Work out the finished part from the listing and answer in its coordinate system (mm). Give positions to 0.01 mm unless a question says otherwise; leave off trailing zeros. Order: outer loops, then holes, each group sorted by start corner. A loop starts at its lowest first (then second) coordinate and runs counter-clockwise, first axis right, second up. Notation, with made-up numbers: (-9, -23) - (23, -23) arc R16 cw to (23, -4) - close; hole circle Ø6 at (54.5, -15.75). An arc over 180 degrees is marked (long way). Put each result on its own line as item: value.
```python
from build123d import *

# Parameters (mm, degrees)
F0_R     = 300
F0_R_2   = 2.25
F0_R_3   = 50
F1_DEPTH = 18


with BuildPart() as f1:
    # F0 (on Top) → F1 (new body)
    with BuildSketch(Plane.XY):
        Circle(F0_R)
        with Locations((-65, -80)):
            Circle(F0_R_2, mode=Mode.SUBTRACT)
        with Locations((-40, -80)):
            Circle(F0_R_2, mode=Mode.SUBTRACT)
        with Locations((40, -80)):
            Circle(F0_R_2, mode=Mode.SUBTRACT)
        with Locations((65, -80)):
            Circle(F0_R_2, mode=Mode.SUBTRACT)
        with Locations((-65, 270)):
            Circle(F0_R_2, mode=Mode.SUBTRACT)
        with Locations((-40, 270)):
            Circle(F0_R_2, mode=Mode.SUBTRACT)
        Circle(F0_R_3, mode=Mode.SUBTRACT)
        with Locations((40, 270)):
            Circle(F0_R_2, mode=Mode.SUBTRACT)
        with Locations((65, 270)):
            Circle(F0_R_2, mode=Mode.SUBTRACT)
    extrude(amount=F1_DEPTH)


solid = f1.part
```
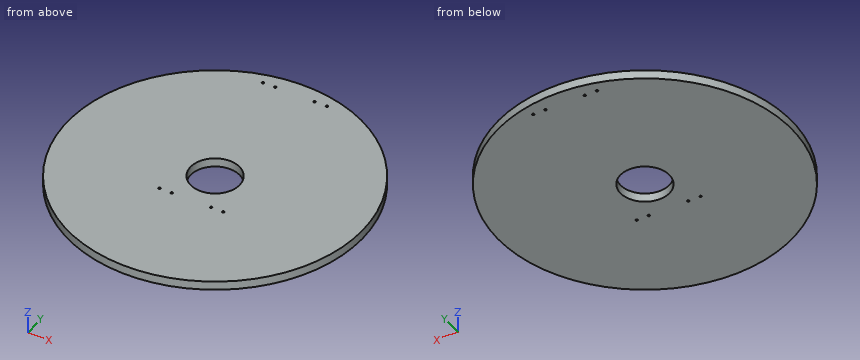
(1) Straight lines are drawn through the part: line 1 (Y direction, x = -40, z = 12.75); line 2 (Y direction, x = 65, z = 9.5); line 3 (Y direction, x = -42.5, z = 9.25). For each, find the intervals that lie inside material, in ascending order.
Geometry check:
line 1: y = -297.32 to -82.25, -77.75 to -30, 30 to 267.75, 272.25 to 297.32
line 2: y = -292.87 to -82.25, -77.75 to 267.75, 272.25 to 292.87
line 3: y = -296.97 to -26.34, 26.34 to 296.97
(2) Section D-D, the plane x = -115.5 is taken. Write down the section's boundary in (y, z), then the cut area to 3 significant figures.
Geometry check:
outline: (-276.87, 0) - (276.87, 0) - (276.87, 18) - (-276.87, 18) - close
area: 9,970 mm²
(3) Section C-C, the plane z = 5.75 is taken. Count the separate pieces of the cut face and the enclosed holes in it, then the cut area to 3 significant figures.
Geometry check:
separate pieces: 1
enclosed holes: 9
area: 275,000 mm²
(4) Section A-A, the plane y = 0 is taken. Write down the section's boundary in (x, z).
Geometry check:
outline: (-300, 0) - (-50, 0) - (-50, 18) - (-300, 18) - close; (50, 0) - (300, 0) - (300, 18) - (50, 18) - close
(5) Given pin 1 (2 mm diameter, centred on x = 190, z = 4.5, fed in from -Y); pin 2 (1 mm diameter, centred on x = -96, z = 16, fed in from +Y); pin 3 (10 mm diameter, centred on y = 138, z = 6.5, fed in from -X), each flat-ended and moving along its own axis, determine where each tip first touches the part or whether it passes through.
Geometry check:
pin 1: stops at y = -232.98
pin 2: stops at y = 284.39
pin 3: stops at x = -268.91
